Check sheet for the drawn part. Datum: minimum x, y, z corner. Units: mm. A direction names the side the tool comes from. Coordinates: 2 decimals unless noted, no trailing zeros. Loops run counter-clockwise (first coordinate to the right, second up) from the corner with the lowest first, then second, coordinate; pieces in that order, holes last.
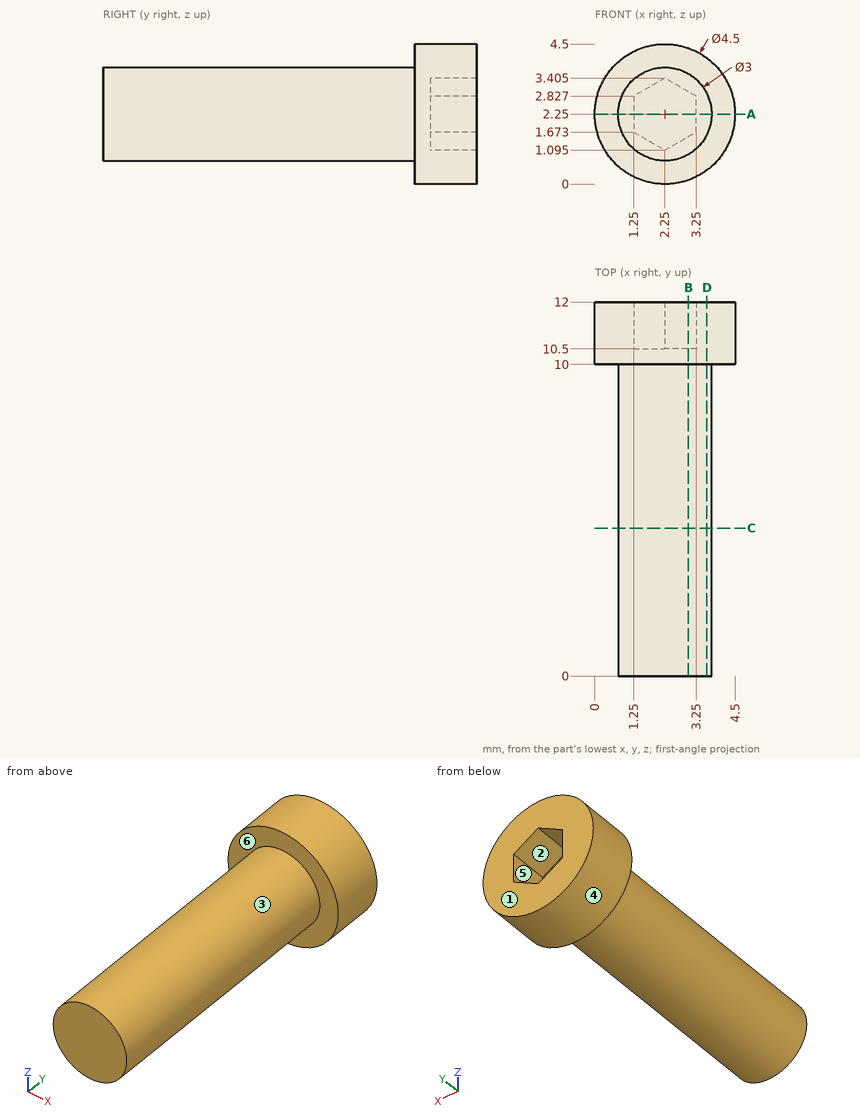
1) Section check C-C on y = 4.75. Enter the section's corners in (x, z).
Answer sheet:
outline: circle Ø3 at (2.25, 2.25)
2) Depth check by flat-ended pin: pin 1 (1 mm diameter, centred on y = 9, z = 1.5, fed in from -X); pin 2 (2 mm diameter, centred on x = 4, y = 6.5, fed in from -Z); pin 3 (0.6 mm diameter, centred on x = 2.5, z = 2.5, fed in from +Y). Enter the tip coordinate at first touch or a pass-through.
Answer sheet:
pin 1: stops at x = 0.77
pin 2: stops at z = 0.95
pin 3: stops at y = 10.5
3) Mould release check, pull along Z, two halves, no side actions. Record for the marked faces 4, 5 and 6: +Z half, -Z half, draft (parallel to the pull), parting line (faces both ways), or undercut.
Answer sheet:
face 4: parting line
face 5: undercut
face 6: draft
4) Section check A-A on z = 2.25. Enter the section's corners in (x, y).
Answer sheet:
outline: (0, 10) - (0.75, 10) - (0.75, 0) - (3.75, 0) - (3.75, 10) - (4.5, 10) - (4.5, 12) - (3.25, 12) - (3.25, 10.5) - (1.25, 10.5) - (1.25, 12) - (0, 12) - close
5) Section check B-B on x = 3. Enter the section's corners in (y, z).
Answer sheet:
outline: (0, 0.95) - (10, 0.95) - (10, 0.13) - (12, 0.13) - (12, 1.53) - (10.5, 1.53) - (10.5, 2.97) - (12, 2.97) - (12, 4.37) - (10, 4.37) - (10, 3.55) - (0, 3.55) - close
6) Set-up check for the marked faces 1, 2 and 3: record each of +Z, -Z, +X, -X, +Y, -Y from which the full face is reachable in a straight line by a thin tool's end or side.
Answer sheet:
face 1: +Z, -Z, +X, -X, +Y
face 2: +Y
face 3: -Y
7) Scan lines: line 1 (Y direction, x = 1.4, z = 2.7); line 2 (Z direction, x = 3.1, y = 8) (1 decimal); line 3 (X direction, y = 2, z = 3.3). Record each from-to range of solid material in increasing order.
Answer sheet:
line 1: y = 0 to 10.5
line 2: z = 1 to 3.5
line 3: x = 1.18 to 3.32
8) Section check D-D on x = 3.6. Enter the section's corners in (y, z).
Answer sheet:
outline: (0, 1.6) - (10, 1.6) - (10, 0.45) - (12, 0.45) - (12, 4.05) - (10, 4.05) - (10, 2.9) - (0, 2.9) - close
